Geometry check sheet. Reference: drawing and pictorial views, mm from the part's lowest x, y, z. Round coordinates to 2 decimals unless told otherwise and drop trailing zeros. Write each loop counter-clockwise with the first axis right and the second up, starting at its lowest first coordinate (ties: lowest second). Pieces come first, ordered by that corner, then holes. Notation, with made-up numbers: (33.5, 31.25) -> (39.5, 31.25) arc R21 cw to (39.5, 57.25) -> close; hole circle Ø9 at (43.25, 53). An arc over 180 degrees is marked (long way). Answer as a JSON object with one key per item and string values. Group by question number.
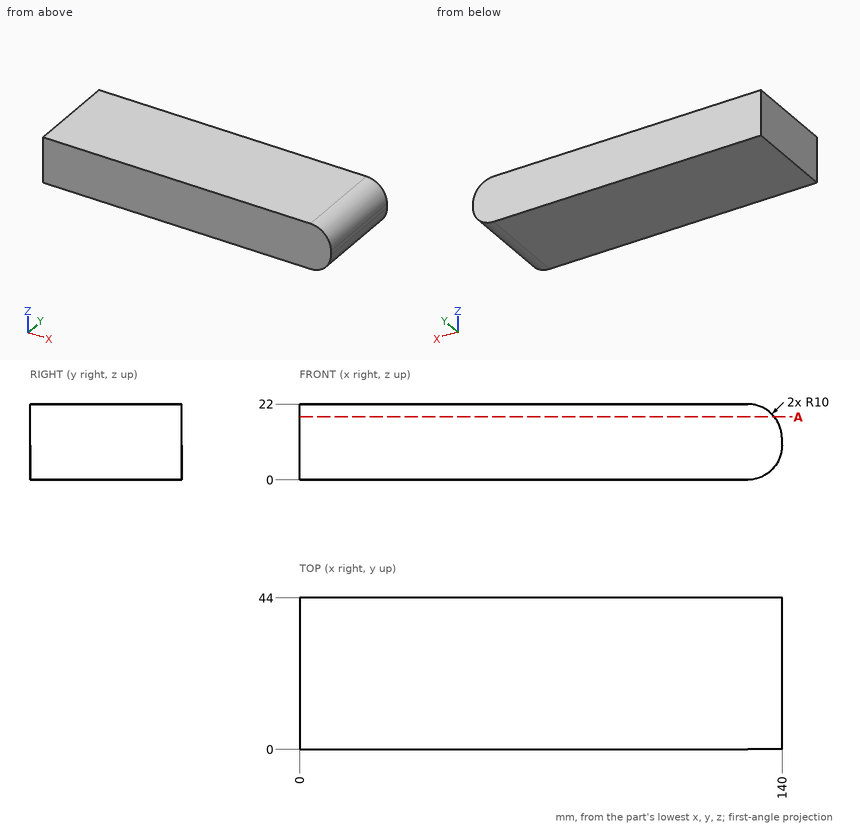
(1) Go/stop test with a flat-tipped pin: pin 1 Ø1.5 at (y, z) = (14.5, 7) entering from +X. Record where the tip stops, or that it passes through.
(2) Section check A-A on z = 18.25. Record the cut outline in (x, y), then the cut area to 3 significant figures.
(3) Scan lines: line 1 along Z through (x, y) = (130.5, 9); line 2 along X through (y, z) = (36, 7.5); line 3 along X through (y, z) = (18.5, 3.5). Record each from-to range of solid material in increasing order.
Data:
{
 "1": {"pin 1": "stops at x = 139.74"},
 "2": {"outline": "(0, 0) -> (137.81, 0) -> (137.81, 44) -> (0, 44) -> close", "area": "6,060 mm²"},
 "3": {"line 1": "z = 0.01 to 21.99", "line 2": "x = 0 to 139.68", "line 3": "x = 0 to 137.6"}
}
